Design review of the part built by this model. Coordinates are the model's own, in mm. A direction names the side the tool comes from. Coordinates: 2 decimals unless noted, no trailing zeros. Loops run counter-clockwise (first coordinate to the right, second up) from the corner with the lowest first, then second, coordinate; pieces in that order, holes last.
Q1. Add section B-B on x = -8.5. Give the boundary of the cut face in (y, z), and give its area (3 significant figures).
Q2. Add section D-D on z = 29.5. Give the boundary of the cut face in (x, y), and give its area (4 significant figures).
Q3. Add section A-A on z = 102. Give the boundary of the cut face in (x, y), and give its area (4 significant figures).
Q4. Wall thickness on probe 1 along Z at (x, y) = (-8.5, 24.95); probe 2 along X at (y, z) = (-7, 5); probe 3 along X at (y, z) = (24, 15): over which ranges is each line inside the solid? List them lowest first.
Q5. Draft analysis for pull direction Y (two halves, no side actions). For faces 1 (the face through (9.93, -11.39, 3.94)), 2 (the face through (0, 25.5, 54)), 3 (the face through (-8.292, 24.232, 100.414)), 4 (the face through (0, -4.5, 4)), state which applies: released by +Y, released by -Y, zero draft, split by the parting line, or undercut.
Q6. Add section C-C on y = 0.5. Give the boundary of the cut face in (x, z).
Q7. Machinability: for faces 5 (the face through (0, 23, 58)), 6 (the face through (0, -10, 4)), which of the approach directions +Z, -Z, +X, -X, +Y, -Y give a long, thin tool a straight path to every point of the face, cutting with its end or side? Answer none if there is none.
Q8. For P1, Ø8, axis at x = 3, z = 22, coming from the -Y side; P2, Ø9, axis at x = 0, y = 0.5, coming from the +Z side; P3, Ø6, axis at y = 18, z = 36, coming from the +X side, all flat-tipped, find the tip position at first contact; note any pin that passes through.
```python
from build123d import *

# Parameters (mm, degrees)
BOSS_EXTRUDE1_DEPTH  = 8
BOSS_EXTRUDE3_DEPTH  = 109
M3_CLEARANCE_SLOT1_D = 3.2


with BuildPart() as part:
    # Sketch1 → Boss-Extrude1 (new body)
    with BuildSketch(Plane.XY):
        with BuildLine():
            Line((15, 23), (-15, 23))
            Line((-15, 23), (-15, -7))
            Line((-15, -7), (-5, -15.660254038))
            ThreePointArc((-5, -15.660254038), (0, -17), (5, -15.660254038))
            Line((5, -15.660254038), (15, -7))
            Line((15, -7), (15, 23))
        make_face()
        with BuildLine():
            Line((1.658312395, -4.5), (-1.658312395, -4.5))
            ThreePointArc((-1.658312395, -4.5), (0, -10), (1.658312395, -4.5))
        make_face(mode=Mode.SUBTRACT)
    extrude(amount=BOSS_EXTRUDE1_DEPTH)

    # Sketch1<5> → Boss-Extrude3 (add)
    with BuildSketch(Plane.XY):
        Polygon((-12.5, 25.5), (12.5, 25.5), (15, 23), (-15, 23), align=None)
    extrude(amount=BOSS_EXTRUDE3_DEPTH)

    # M3 Clearance Slot1 (through all)
    with Locations(Plane(origin=(0, 25.5, 0), x_dir=(1, 0, 0), z_dir=(0, 1, 0))):
        with Locations((-8.5, -15), (8.5, -15), (-8.5, -102), (8.5, -102)):
            Hole(M3_CLEARANCE_SLOT1_D / 2)


solid = part.part
```
Entries:
1. outline: (-12.63, 0) - (25.5, 0) - (25.5, 13.4) - (23, 13.4) - (23, 8) - (-12.63, 8) - close; (23, 16.6) - (25.5, 16.6) - (25.5, 100.4) - (23, 100.4) - close; (23, 103.6) - (25.5, 103.6) - (25.5, 109) - (23, 109) - close
1. area: 542 mm2
2. outline: (-15, 23) - (15, 23) - (12.5, 25.5) - (-12.5, 25.5) - close
2. area: 68.75 mm2
3. outline: (-15, 23) - (-10.1, 23) - (-10.1, 25.5) - (-12.5, 25.5) - close; (-6.9, 23) - (6.9, 23) - (6.9, 25.5) - (-6.9, 25.5) - close; (10.1, 23) - (15, 23) - (12.5, 25.5) - (10.1, 25.5) - close
3. area: 52.75 mm2
4. probe 1: z = 0 to 13.4, 16.6 to 100.4, 103.6 to 109
4. probe 2: x = -15 to -3, 3 to 15
4. probe 3: x = -14 to -10.1, -6.9 to 6.9, 10.1 to 14
5. face 1: released by -Y
5. face 2: released by +Y
5. face 3: zero draft
5. face 4: undercut
6. outline: (-15, 0) - (15, 0) - (15, 8) - (-15, 8) - close
7. face 5: +Z, +X, -X, -Y
7. face 6: +Z, -Z
8. P1: stops at y = 23
8. P2: stops at z = 8
8. P3: passes through
